Input: part model. Units: mm. Frame: model coordinates. A direction names the side the tool comes from. Coordinates: 2 decimals unless noted, no trailing zeros. Loops run counter-clockwise (first coordinate to the right, second up) from the corner with the lowest first, then second, coordinate; pieces in that order, holes last. Notation, with made-up numbers: (8.25, 86.25) -> (38.25, 86.25) arc R16 cw to (38.25, 95.25) -> close; hole circle Ø1 at (45.25, 55). An arc over 180 degrees is marked (long way). Answer as a JSON object with one key per item and string values.
Autodesk Inventor part; units mm, degrees
ref_plane "YZ Plane" through (0, 0, 0) normal (1, 0, 0) x (0, 1, 0)
ref_plane "XZ Plane" through (0, 0, 0) normal (0, 1, 0) x (-1, 0, 0)
ref_plane "XY Plane" through (0, 0, 0) normal (0, 0, 1) x (1, 0, 0)
sketch "Sketch1" plane through (0, 0, 0) normal (0, 1, 0) x (-1, 0, 0)
  circle A0 centre (0, 0) radius 32
  dimension "d0" = 64
extrude "Extrusion1" add sketch "Sketch1" along normal blind 2
sketch "Sketch2" plane through (0, 0, 0) normal (0, -1, 0) x (1, 0, 0)
  circle A0 centre (0, 0) radius 20.75
  circle A1 centre (0, 0) radius 20
  dimension "d3" = 41.5
  dimension "d4" = 40
extrude "Extrusion2" add sketch "Sketch2" along normal blind 2
sketch "Sketch4" plane through (0, 0, 0) normal (0, -1, 0) x (1, 0, 0)
  circle A0 centre (19, 19) radius 2.75
  point P0 (0, 0)
  dimension "d9" = 5.5
  dimension "d10" = 19
  dimension "d11" = 19
extrude "Extrusion4" add sketch "Sketch4" along normal blind 6.5
pattern_circular "Circular Pattern1" count 4 over 360 about axis through (0, -10, 0) along (0, 1, 0) of "Extrusion4"
sketch "Sketch5" plane through (0, 2, 0) normal (0, 1, 0) x (1, 0, 0)
  line L0 (-12.25, 12.25) -> (12.25, 12.25)
  line L1 (12.25, 12.25) -> (12.25, -12.25)
  line L2 (12.25, -12.25) -> (-12.25, -12.25)
  line L3 (-12.25, -12.25) -> (-12.25, 12.25)
  line L4 (-12.25, 12.25) -> (12.25, -12.25) construction
  line L5 (12.25, 12.25) -> (-12.25, -12.25) construction
  point P0 (0, 0)
  dimension "d17" = 24.5
  dimension "d18" = 24.5
extrude "Extrusion5" add sketch "Sketch5" along normal blind 2
sketch "Sketch6" plane through (0, 4, 0) normal (0, 1, 0) x (1, 0, 0)
  line L0 (12.25, 12.25) -> (-12.25, 12.25)
  line L1 (-12.25, 12.25) -> (-12.25, -12.25)
  line L2 (-12.25, -12.25) -> (12.25, -12.25)
  line L3 (12.25, -12.25) -> (12.25, 12.25)
  circle A0 centre (0, 0) radius 10
  dimension "d21" = 20
extrude "Extrusion6" cut sketch "Sketch6" against normal through all contours A0
fillet "Fillet1" radius 2 1 edges at (-10, 0, 0)
properties part number "pot_base_adapter2"
1. Access query for faces 5 (the face through (-19, -6.5, 19)), 6 (the face through (12.25, 3, 0)), 7 (the face through (18.642, -3.204, 16.273)), 8 (the face through (6.94, 0.99, 31.24)), 9 (the face through (-12.25, 3, 0)). Directions: +Z, -Z, +X, -X, +Y, -Y. A direction counts if a zero-diameter tool reaches every point of the face in a straight line with its end or side. Return the directions, or none.
Reply:
{"face 5": "+Z, -Z, +X, -X, -Y", "face 6": "+Z, -Z, +X, +Y", "face 7": "-Y", "face 8": "+Y, -Y", "face 9": "+Z, -Z, -X, +Y"}
2. Line query: line 1 along Z through (x, y) = (0, -0.45); line 2 along X through (y, z) = (3.45, 0). Output: solid intervals per line, ascending.
Reply:
{"line 1": "z = -20.75 to -20, 20 to 20.75", "line 2": "x = -12.25 to -10, 10 to 12.25"}
3. Section query B-B (y = -4.5). Return loops of the section in (x, z), plus the area to 3 significant figures.
Reply:
{"outline": "circle Ø5.5 at (-19, -19); circle Ø5.5 at (-19, 19); circle Ø5.5 at (19, -19); circle Ø5.5 at (19, 19)", "area": "95.0 mm2"}
4. Mould query, pull axis Z, two halves, no side actions, for faces 1 (the face through (-19, -6.5, -19)), 2 (the face through (-4.336, -0.986, 19.524)), 3 (the face through (0, 3, 12.25)), 4 (the face through (0, 3, -12.25)). Classes: pulls with the +Z half, pulls with the -Z half, needs draft (parallel to the pull), parting line crosses it, or undercut.
Reply:
{"face 1": "needs draft", "face 2": "undercut", "face 3": "pulls with the +Z half", "face 4": "pulls with the -Z half"}
5. Section query C-C (x = 15). Return loops of the section in (y, z), plus the area to 3 significant figures.
Reply:
{"outline": "(-2, -14.34) -> (0, -14.34) -> (0, -28.27) -> (2, -28.27) -> (2, 28.27) -> (0, 28.27) -> (0, 14.34) -> (-2, 14.34) -> (-2, 13.23) -> (0, 13.23) -> (0, -13.23) -> (-2, -13.23) -> close", "area": "118 mm2"}
6. Section query A-A (z = 0). Return loops of the section in (x, y).
Reply:
{"outline": "(-32, 0) -> (-20.75, 0) -> (-20.75, -2) -> (-20, -2) -> (-20, 0) -> (-12, 0) arc R2 ccw to (-10, 2) -> (-10, 4) -> (-12.25, 4) -> (-12.25, 2) -> (-32, 2) -> close; (10, 2) arc R2 ccw to (12, 0) -> (20, 0) -> (20, -2) -> (20.75, -2) -> (20.75, 0) -> (32, 0) -> (32, 2) -> (12.25, 2) -> (12.25, 4) -> (10, 4) -> close"}
7. Section query D-D (z = 19). Return loops of the section in (x, y) (3 decimals), plus the area to 3 significant figures.
Reply:
{"outline": "(-25.749, 0) -> (-21.75, 0) -> (-21.75, -6.5) -> (-16.25, -6.5) -> (-16.25, 0) -> (-8.34, 0) -> (-8.34, -2) -> (-6.245, -2) -> (-6.245, 0) -> (6.245, 0) -> (6.245, -2) -> (8.34, -2) -> (8.34, 0) -> (16.25, 0) -> (16.25, -6.5) -> (21.75, -6.5) -> (21.75, 0) -> (25.749, 0) -> (25.749, 2) -> (-25.749, 2) -> close", "area": "183 mm2"}
8. Pin query (flat end, axial travel): P1, Ø6, axis at y = -1, z = 5.5, coming from the +X side; P2, Ø4, axis at x = -23.5, y = -2.5, coming from the +Z side; P3, Ø0.6, axis at y = 3, z = 6, coming from the +X side; P4, Ø4, axis at x = 4, y = -5.5, coming from the +Z side. Return the tip coordinate at first contact, or that it passes through.
Reply:
{"P1": "stops at x = 31.89", "P2": "stops at z = 20.15", "P3": "stops at x = 12.25", "P4": "passes through"}
